Could you check a few things on this drawing? It's one solid part, dimensions in mm from its lowest x, y, z. Round coordinates to 2 decimals unless told otherwise and drop trailing zeros. Write each loop counter-clockwise with the first axis right and the second up, starting at its lowest first coordinate (ties: lowest second). Pieces come first, ordered by that corner, then holes. Notation, with made-up numbers: (4.5, 26) -> (47.5, 26) arc R17 cw to (47.5, 36) -> close; hole circle Ø1 at (84, 30.25). An arc over 180 degrees is marked (long way). Put each result on its own line as item: value. Start each with the question number.
1) I want a section at D-D, the plane z = 6. List the corners of the cut face in (x, y) for me, then the cut area to 3 significant figures.
2) I want a section at A-A, the plane y = 38.1. List the corners of the cut face in (x, z) for me, then the cut area to 3 significant figures.
3) We'd pull the mould along X, two halves only. Please class the marked faces 1, 2 and 3: released by +X, released by -X, zero draft, split by the parting line, or undercut.
4) If I drill on line 1 along X through (y, z) = (38, 4); line 2 along Z through (x, y) = (73, 45.5), over which ranges is the centre line in solid material (lowest first)? Write a range as [from, to].
5) I want a section at C-C, the plane z = 33. Give the number of separate pieces and of enclosed holes in the cut face, then the cut area to 3 significant figures.
6) Will these pins go through, and if not, where does the flat tip stop? P1, Ø1, axis at x = 15, z = 24.5, coming from the -Y side; P2, Ø5, axis at x = 30.5, y = 58, coming from the -Z side; P3, Ø12, axis at x = 59.5, z = 12.5, coming from the +Y side; P4, Ø3, axis at y = 63.5, z = 13.5, coming from the +X side (1 decimal).
7) I want a section at B-B, the plane x = 38.1. List the corners of the cut face in (y, z) for me.
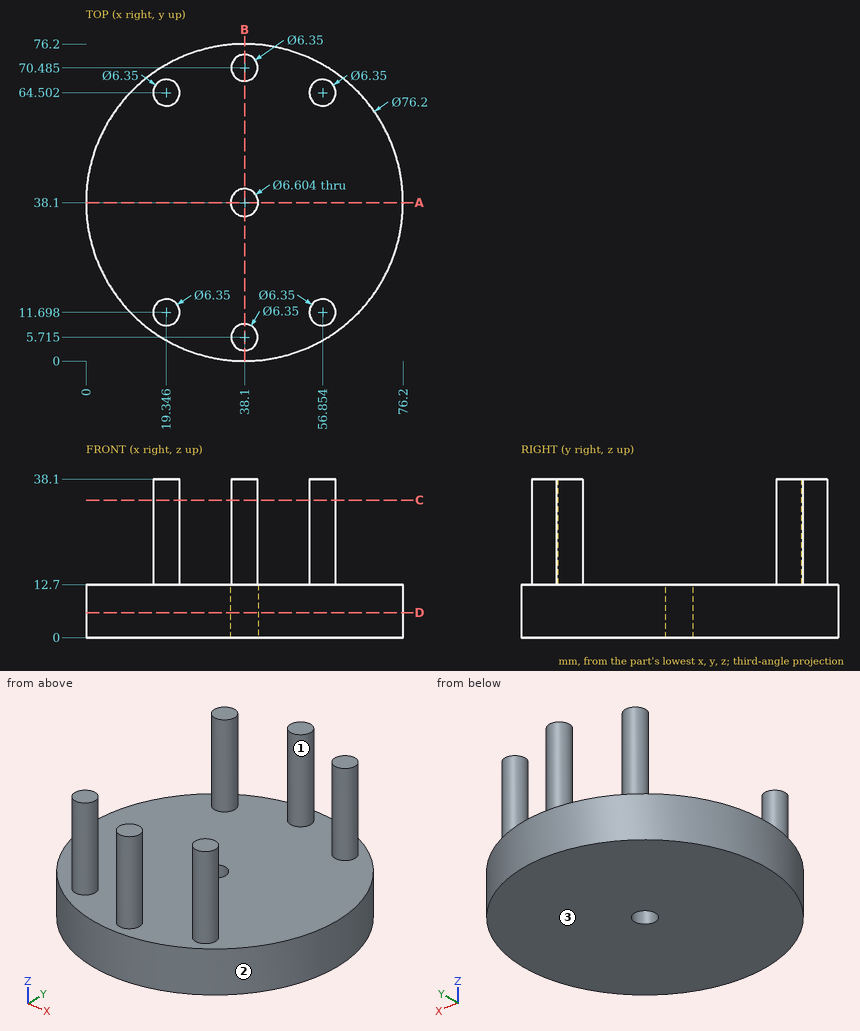
Findings:
1. outline: circle Ø76.2 at (38.1, 38.1); hole circle Ø6.6 at (38.1, 38.1)
1. area: 4,530 mm2
2. outline: (0, 0) -> (34.8, 0) -> (34.8, 12.7) -> (0, 12.7) -> close; (41.4, 0) -> (76.2, 0) -> (76.2, 12.7) -> (41.4, 12.7) -> close
2. area: 884 mm2
3. face 1: undercut
3. face 2: split by the parting line
3. face 3: zero draft
4. line 1: x = [0, 34.8], [41.4, 76.2]
4. line 2: z = [0, 12.7]
5. separate pieces: 6
5. enclosed holes: 0
5. area: 190 mm2
6. P1: passes through
6. P2: stops at z = 0
6. P3: stops at y = 72.95
6. P4: stops at x = 67.6
7. outline: (0, 0) -> (34.8, 0) -> (34.8, 12.7) -> (8.89, 12.7) -> (8.89, 38.1) -> (2.54, 38.1) -> (2.54, 12.7) -> (0, 12.7) -> close; (41.4, 0) -> (76.2, 0) -> (76.2, 12.7) -> (73.66, 12.7) -> (73.66, 38.1) -> (67.31, 38.1) -> (67.31, 12.7) -> (41.4, 12.7) -> close
